from build123d import *

# Parameters (mm, degrees)
F2_DEPTH = 30
F3_W     = 630
F3_H     = 25
F4_DEPTH = 600
F5_W     = 447.4647887324
F5_H     = 18
F6_DEPTH = 500
F7_W     = 50.4934979443
F7_H     = 50
F8_DEPTH = 500


with BuildPart() as f2:
    # F1 (on offset) → F2 (new body)
    with BuildSketch(Plane.YZ.offset(500)):
        Polygon((-600, 50), (-600, 0), (0, 0), (0, 50), (-150, 1115), (-600, 1115), (-450, 50), align=None)
        Polygon((-50.4934979443, 50), (-373.9965395023, 50), (-183.0022161165, 990.8118990221), align=None, mode=Mode.SUBTRACT)
        Polygon((-409.9555303624, 124.1881009779), (-542.4642485345, 1065), (-218.9612069765, 1065), align=None, mode=Mode.SUBTRACT)
    extrude(amount=F2_DEPTH)

    # F3 (on Front) → F4 (join)
    with BuildSketch(Plane.XZ):
        with Locations((315, 1127.5)):
            Rectangle(F3_W, F3_H)
    extrude(amount=F4_DEPTH)

    # F5 (on Right) → F6 (join, through all)
    with BuildSketch(Plane.YZ):
        with Locations((-345.5633802817, 906)):
            Rectangle(F5_W, F5_H)
        with Locations((-303.7323943662, 609)):
            Rectangle(F5_W, F5_H)
        with Locations((-247.3943661972, 209)):
            Rectangle(F5_W, F5_H)
    extrude(amount=F6_DEPTH)

    # F7 (on Right) → F8 (join, through all)
    with BuildSketch(Plane.YZ):
        with Locations((-25.2467489722, 25)):
            Rectangle(F7_W, F7_H)
    extrude(amount=F8_DEPTH)

    # F9: F2 across plane


with BuildPart() as f2_1:
    add(f2.part)
    add(f2.part.mirror(Plane.YZ))


solid = f2_1.part
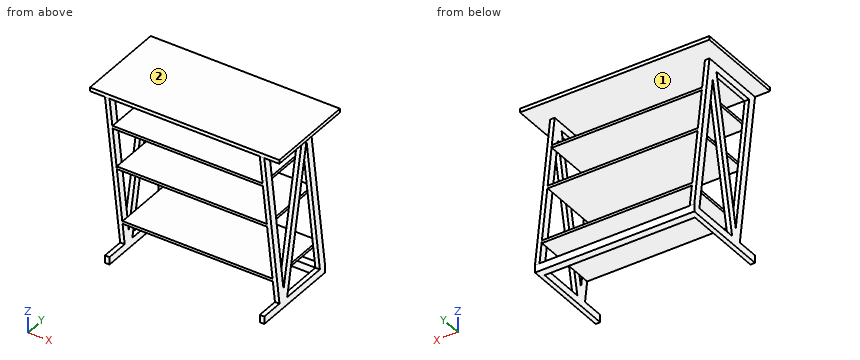
The listing builds one solid part. Answer for the finished solid, in the listing's coordinates (mm). Face numbers are marked on the shaded views. Coordinates: 2 decimals unless noted, no trailing zeros. Loops run counter-clockwise (first coordinate to the right, second up) from the corner with the lowest first, then second, coordinate; pieces in that order, holes last. Notation, with made-up numbers: M 77.5,28 L 101.5,28 A8 ccw 101.5,42 Z; hole C -7,25.5 d3. An arc over 180 degrees is marked long. Answer in a Markdown table with one row per item.
1) Find section A-A (x = 48). Determine the outline of the cut face in (y, z).
Answers below:
| item | result |
|---|---|
| outline | M -600,1115 L 0,1115 L 0,1140 L -600,1140 Z; M -569.3,897 L -121.83,897 L -121.83,915 L -569.3,915 Z; M -527.46,600 L -80,600 L -80,618 L -527.46,618 Z; M -471.13,200 L -23.66,200 L -23.66,218 L -471.13,218 Z; M -50.49,0 L 0,0 L 0,50 L -50.49,50 Z |
2) Determine the mould class of the marked faces 1 and 2 for opening direction Z: released by +Z, released by -Z, zero draft, split by the parting line, or undercut.
Answers below:
| item | result |
|---|---|
| face 1 | undercut |
| face 2 | released by +Z |
3) Find section B-B (z = 778). Determine the outline of the cut face in (x, y).
Answers below:
| item | result |
|---|---|
| outline | M -530,-552.54 L -500,-552.54 L -500,-502.04 L -530,-502.04 Z; M -530,-277.23 L -500,-277.23 L -500,-226.21 L -530,-226.21 Z; M -530,-153.03 L -500,-153.03 L -500,-102.54 L -530,-102.54 Z; M 500,-552.54 L 530,-552.54 L 530,-502.04 L 500,-502.04 Z; M 500,-277.23 L 530,-277.23 L 530,-226.21 L 500,-226.21 Z; M 500,-153.03 L 530,-153.03 L 530,-102.54 L 500,-102.54 Z |
4) Given pin 1 (4 mm diameter, centred on x = -429.5, y = -92, fed in from -Z); pin 2 (5.5 mm diameter, centred on y = -196.5, z = 613.5, fed in from -X); pin 3 (5.5 mm diameter, centred on x = 117.5, z = 903.5, fed in from +Y), each flat-ended and moving along its own axis, determine where each tip first touches the part or whether it passes through.
Answers below:
| item | result |
|---|---|
| pin 1 | z = 200 |
| pin 2 | x = -500 |
| pin 3 | y = -121.83 |
5) Find section C-C (x = -546). Determine the outline of the cut face in (y, z), then the cut area to 3 significant figures.
Answers below:
| item | result |
|---|---|
| outline | M -600,1115 L 0,1115 L 0,1140 L -600,1140 Z |
| area | 15,000 mm^2 |
6) Find the intervals of material crossed by probe 1 along Z at (x, y) = (418.5, -211.5); probe 2 along Z at (x, y) = (-11, -107.5); probe 3 along Z at (x, y) = (-168.5, -58), in increasing order.
Answers below:
| item | result |
|---|---|
| probe 1 | 200 to 218, 600 to 618, 897 to 915, 1115 to 1140 |
| probe 2 | 200 to 218, 600 to 618, 1115 to 1140 |
| probe 3 | 200 to 218, 1115 to 1140 |
